Model file for the job. Use its own axes, mm. Face numbers are marked on the shaded views. Round coordinates to 2 decimals unless told otherwise and drop trailing zeros. Order: outer loops, then holes, each group sorted by start corner. A loop starts at its lowest first (then second) coordinate and runs counter-clockwise, first axis right, second up. Notation, with made-up numbers: (80.5, 29.5) - (116.5, 29.5) arc R17 ccw to (116.5, 44.5) - close; hole circle Ø9 at (-4, -24.75). An arc over 180 degrees is marked (long way). Put each result on its own line as item: value. Start each with the question number.
Item 1: Pin check, flat tips, straight feed: pin 1 Ø1 at (x, z) = (22.5, 3.5) entering from +Y (3 decimals); pin 2 Ø20.5 at (x, y) = (16, -29.5) entering from +Z; pin 3 Ø0.6 at (x, z) = (5, 3.5) entering from -Y (3 decimals). Stop position of each tip, or through.
Item 2: Saw through at C-C on z = 3.65. List the corners of the cut face in (x, y).
Item 3: Saw through at B-B on x = 11. List the corners of the cut face in (y, z).
Item 4: Probe probe 1 along Y at (x, z) = (8, 2.55); probe 2 along Z at (x, y) = (19, -7); probe 3 along Y at (x, z) = (25, 3.45). List the from-to ranges inside material, lowest first.
Item 5: Mould opens along Y. For the marked faces 1 and 2 say: pulls with the +Y half, pulls with the -Y half, needs draft (parallel to the pull), parting line crosses it, or undercut.
Item 6: Saw through at A-A on y = -51.5. List the corners of the cut face in (x, z), plus the area to 4 significant figures.
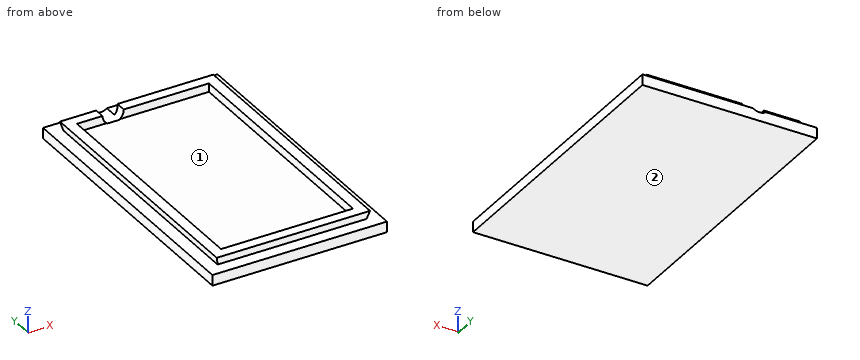
Autodesk Inventor part; units mm, degrees
ref_plane "YZ Plane" through (0, 0, 0) normal (1, 0, 0) x (0, 1, 0)
ref_plane "XZ Plane" through (0, 0, 0) normal (0, 1, 0) x (-1, 0, 0)
ref_plane "XY Plane" through (0, 0, 0) normal (0, 0, 1) x (1, 0, 0)
sketch "Sketch1" plane through (0, 0, 0) normal (0, 0, 1) x (1, 0, 0)
  line L0 (0, 0) -> (36, 0)
  line L1 (36, 0) -> (36, -62)
  line L2 (36, -62) -> (0, -62)
  line L3 (0, -62) -> (0, 0)
  line L4 (-2.5, 2.5) -> (38.5, 2.5)
  line L5 (38.5, 2.5) -> (38.5, -64.5)
  line L6 (38.5, -64.5) -> (-2.5, -64.5)
  line L7 (-2.5, -64.5) -> (-2.5, 2.5)
  dimension "d0" = 36
  dimension "d1" = 62
  dimension "d2" = 2.5
extrude "Extrusion1" add sketch "Sketch1" along normal blind 2.5 contours L0 L1 L2 L3 | L4 L5 L6 L7
sketch "Sketch2" plane through (0, 0, 2.5) normal (0, 0, 1) x (1, 0, 0)
  line L0 (38.5, 2.5) -> (-2.5, 2.5)
  line L1 (-2.5, 2.5) -> (-2.5, -64.5)
  line L2 (-2.5, -64.5) -> (38.5, -64.5)
  line L3 (38.5, -64.5) -> (38.5, 2.5)
  line L4 (0, 0) -> (36, 0)
  line L5 (36, 0) -> (36, -62)
  line L6 (36, -62) -> (0, -62)
  line L7 (0, -62) -> (0, 0)
  line L8 (2.5, -2.5) -> (33.5, -2.5)
  line L9 (33.5, -2.5) -> (33.5, -59.5)
  line L10 (33.5, -59.5) -> (2.5, -59.5)
  line L11 (2.5, -59.5) -> (2.5, -2.5)
  point P0 (0, 0)
  dimension "d5" = 2.5
  dimension "d6" = 2.5
extrude "Extrusion2" add sketch "Sketch2" along normal blind 2 contours L4 L5 L6 L7
sketch "Sketch3" plane through (0, -62, 2.5) normal (-1, 0, 0) x (0, 0, 1)
  line L0 (0, 62) -> (2, 62)
  line L1 (0, 62) -> (0, 61.5)
  line L2 (0, 64.5) -> (0, -2.5)
  line L3 (2, 62) -> (2, 0)
  line L4 (0, 61.5) -> (2, 62)
  line L5 (2, 62) -> (0, 62)
  line L6 (0, 0) -> (0, 0.5)
  line L7 (0, 0) -> (0, 62)
  line L8 (0, 0.5) -> (2, 0)
  line L9 (0, 0) -> (2, 0)
  line L10 (2, 0) -> (0, 0)
  point P0 (-2.5, 62)
  dimension "d9" = 0.5
  dimension "d10" = 0.5
sketch "Sketch4" plane through (0, 0, 2.5) normal (0, 1, 0) x (1, 0, 0)
  line L0 (36, 0) -> (36, -2)
  line L1 (36, -2) -> (36, 0)
  line L2 (36, 0) -> (35.5, 0)
  line L3 (36, 0) -> (0, 0)
  line L4 (35.5, 0) -> (36, -2)
  line L5 (0, 0) -> (0, -2)
  line L6 (0, -2) -> (0, 0)
  line L7 (0, 0) -> (0.5, 0)
  line L8 (0.5, 0) -> (0, -2)
  point P0 (0, 2.5)
  dimension "d13" = 0.5
  dimension "d14" = 0.5
extrude "Extrusion3" cut sketch "Sketch3" against normal through all contours L0 L4 L1 | L9 L2 L8
extrude "Extrusion4" cut sketch "Sketch4" against normal through all
sketch "Sketch5" plane through (-2.5, 2.5, 0) normal (0, 1, 0) x (1, 0, 0)
  line L0 (5, -4.5) -> (36, -4.5)
  line L1 (20.5, -4.5) -> (13.5, -4.5)
  circle A0 centre (13.5, -4.5) radius 2.5
  point P0 (2.5, 0)
  dimension "d17" = 7
  dimension "d18" = 5
extrude "Extrusion5" cut sketch "Sketch5" against normal blind 5
fillet "Fillet1" radius 0.25 1 edges at (11, -2.5, 2.5)
properties part number "feeder_encolsure_lid"
Results found:
1. pin 1: stops at y = -0.125
1. pin 2: stops at z = 2.5
1. pin 3: stops at y = -61.825
2. outline: (0.21, -61.79) - (35.79, -61.79) - (35.79, -0.21) - (13.35, -0.21) - (13.35, -2.5) - (33.5, -2.5) - (33.5, -59.5) - (2.5, -59.5) - (2.5, -2.5) - (8.65, -2.5) - (8.65, -0.21) - (0.21, -0.21) - close
3. outline: (-64.5, 0) - (2.5, 0) - (2.5, 2) - (-2.5, 2) - (-2.5, 2.25) arc R0.25 ccw to (-2.75, 2.5) - (-59.5, 2.5) - (-59.5, 4.5) - (-62, 4.5) - (-61.5, 2.5) - (-64.5, 2.5) - close
4. probe 1: y = -61.51 to -59.5, -2.5 to -0.49
4. probe 2: z = 0 to 2.5
4. probe 3: y = -61.74 to -59.5, -2.5 to -0.26
5. face 1: undercut
5. face 2: needs draft
6. outline: (-2.5, 0) - (38.5, 0) - (38.5, 2.5) - (35.5, 2.5) - (36, 4.5) - (33.5, 4.5) - (33.5, 2.5) - (2.5, 2.5) - (2.5, 4.5) - (0, 4.5) - (0.5, 2.5) - (-2.5, 2.5) - close
6. area: 111.5 mm²
